Input: part model. Units: mm. Frame: model coordinates. A direction names the side the tool comes from. Coordinates: 2 decimals unless noted, no trailing zeros. Write each loop counter-clockwise with the first axis right and the second up, starting at its lowest first coordinate (ties: lowest second). Pieces come first, ordered by that corner, then holes. Notation, with made-up numbers: (17, 12.25) - (49, 12.25) arc R25 ccw to (49, 48.25) - close; hole circle Ø2 at (71.25, -22.75). An arc over 180 degrees is marked (long way). Put each result on its own line as item: value. Start each with the question number.
1. Access query for faces 1 (the cylindrical face through (3.16, -0.27, 1.22)), 2 (the cylindrical face through (0.2, -2.35, -0.05)). Directions: +Z, -Z, +X, -X, +Y, -Y. A direction counts if a zero-diameter tool reaches every point of the face in a straight line with its end or side. Return the directions, or none.
2. Cut plane C-C, the plane x = 0.95. Return loops of the section in (y, z), and give its area (3 significant figures).
3. Pin query (flat end, axial travel): pin 1 (1.5 mm diameter, centred on y = 1, z = 1, fed in from -X); pin 2 (1.5 mm diameter, centred on y = -1, z = 1.5, fed in from +X); pin 3 (1.5 mm diameter, centred on x = 1, z = -1.5, fed in from -Y); pin 4 (1 mm diameter, centred on x = 3.5, z = -0.5, fed in from -Y). Return the tip coordinate at first contact, or that it passes through.
4. Cut plane B-B, the plane z = 0. Return loops of the section in (x, y).
5. Cut plane D-D, the plane x = 3.3. Return loops of the section in (y, z), and give its area (3 significant figures).
6. Line query: line 1 (Z direction, x = 4.7, y = 0.4); line 2 (Y direction, x = 1, z = 0); line 3 (Z direction, x = 1.3, y = -0.3). Output: solid intervals per line, ascending.
7. Cut plane A-A, the plane y = 0. Return loops of the section in (x, z).
Autodesk Inventor part; units mm, degrees
ref_plane "Work Plane1" through (33.575, 0, 0) normal (0, 0, -1) x (1, 0, 0)
ref_plane "YZ Plane" through (0, 0, 0) normal (1, 0, 0) x (0, 1, 0)
ref_plane "XZ Plane" through (0, 0, 0) normal (0, 1, 0) x (-1, 0, 0)
sketch "Skizze1" plane through (0, 0, 0) normal (0, 0, 1) x (1, 0, 0)
  line L0 (0, 0) -> (5, 0)
  line L1 (5, 0) -> (5, 1.25)
  line L2 (5, 1.25) -> (2.4, 1.25)
  line L3 (2.4, 1.25) -> (2.1239, 1.25)
  line L4 (2.1239, 1.25) -> (1.5, 1.25)
  line L5 (1.5, 1.25) -> (0.4, 2.35)
  line L6 (0.4, 2.35) -> (0, 2.35)
  line L7 (0, 2.35) -> (0, 0)
  line L8 (2.4, 1.25) -> (1.5, 1.25) construction
  line L9 (-1, 0) -> (6, 0)
  line L10 (0, 2.82) -> (0, -0.47)
  dimension "d0" = 5
  dimension "d1" = 45
  dimension "d2" = 0.2761
  dimension "d3" = 2.6
  dimension "d4" = 1.5
  dimension "d5" = 2.5
  dimension "d6" = 2.5
  dimension "d7" = 4.7
revolve "Körper" add sketch "Skizze1" angle 360 about axis through (0, 0, 0) along (1, 0, 0)
sketch "Skizze2" plane through (0, 0, 0) normal (-1, 0, 0) x (0, 0, 1)
  line L0 (2.35, -0.3) -> (-2.35, -0.3)
  line L1 (-2.35, -0.3) -> (-2.35, 0.3)
  line L2 (-2.35, 0.3) -> (2.35, 0.3)
  line L3 (2.35, 0.3) -> (2.35, -0.3)
  line L4 (0, 0.3) -> (0, -0.3) construction
  line L5 (-2.35, 0) -> (2.35, 0) construction
  line L6 (0, 2.35) -> (0, 0)
  dimension "d15" = 0.6
  dimension "d16" = 4.7
extrude "Loch" cut sketch "Skizze2" against normal blind 0.7
thread "Gewinde"
chamfer "Fase1" distance 0.2761 distance2 0.138 1 edges at (5, -1.25, 0) measured on face at (5, -0.3689, 0.4922)
ref_plane "Work Plane1" through (33.575, 0, 0) normal (0, 0, -1) x (1, 0, 0)
equation "\"d0\" = NLG"
equation "\"d1\" = 0.5 * SEWI"
equation "\"d2\" = GAL"
equation "\"d3\" = GEL"
equation "\"d4\" = KOH"
equation "\"d5\" = BDM"
equation "\"d6\" = GD"
equation "\"d7\" = KOD"
equation "\"d15\" = SBR"
equation "\"d16\" = KOD"
equation "\"d8\" = STI"
equation "\"d10\" = GEL"
equation "\"d12\" = -0.5 * SPD + 0.5 * GD"
equation "\"d13\" = 0.5 * GAL"
equation "\"NLG\" = 5"
equation "\"GAL\" = 0.61345 * PTC"
equation "\"GEL\" = 2.6"
equation "\"KOH\" = 1.5"
equation "\"KOD\" = 4.7"
equation "\"SEWI\" = 90deg"
equation "\"BDM\" = NND"
equation "\"GD\" = NND"
equation "\"SBR\" = 0.6"
equation "\"STI\" = 0.7"
equation "\"SPD\" = NND - 1.2269 * PTC"
equation "\"GUL\" = 0.61345 * PTC"
equation "\"PTC\" = 0.45"
equation "\"EPV\" = 2.75"
equation "\"THREADDIA\" = 2.5"
equation "\"TOA\" = 30deg"
equation "\"NND\" = 2.5"
equation "\"GD1\" = THREADDIA - 1.2269 * PTC"
properties part number "DIN 963 - M2,5 x 5" material "Edelstahl"
Report:
1. face 1: +X
1. face 2: +X, -X, -Y
2. outline: circle Ø3.6 at (0, 0)
2. area: 10.2 mm^2
3. pin 1: stops at x = 0
3. pin 2: stops at x = 4.96
3. pin 3: stops at y = -2.1
3. pin 4: stops at y = -1.25
4. outline: (0, -2.35) - (0.4, -2.35) - (1.5, -1.25) - (4.86, -1.25) - (5, -0.97) - (5, 0.97) - (4.86, 1.25) - (1.5, 1.25) - (0.4, 2.35) - (0, 2.35) - (0, 0.3) - (0.7, 0.3) - (0.7, -0.3) - (0, -0.3) - close
5. outline: circle Ø2.5 at (0, 0)
5. area: 4.91 mm^2
6. line 1: z = -1.18 to 1.18
6. line 2: y = -1.75 to 1.75
6. line 3: z = -1.42 to 1.42
7. outline: (0.7, -2.05) - (1.5, -1.25) - (4.86, -1.25) - (5, -0.97) - (5, 0.97) - (4.86, 1.25) - (1.5, 1.25) - (0.7, 2.05) - close
